from build123d import *

# Parameters (mm, degrees)
F0_R     = 11
F1_DEPTH = 7
F4_DEPTH = 0.4


with BuildPart() as f1:
    # F0 (on Front) → F1 (new body)
    with BuildSketch(Plane.XZ):
        with BuildLine():
            add(Edge.make_bspline(
                [(-90.8271871838, 17.1252166849), (-65.6361619016, 20.1801984156), (-15.2541113371, 26.2901618769), (15.053487254, 66.9980498131), (30.2072865496, 87.3519937812)],
                knots=[0, 0, 0, 0, 0.5, 1, 1, 1, 1], degree=3))
            ThreePointArc((-90.8271871838, 17.1252166849), (-100.7899149472, -0.2167571218), (-90.7526889605, -17.5157193593))
            add(Edge.make_bspline(
                [(-90.7526889605, -17.5157193593), (-65.5487567691, -20.462322529), (-15.1408923865, -26.3555288685), (15.3415164695, -66.9326828214), (30.5827208975, -87.2212597979)],
                knots=[0, 0, 0, 0, 0.5, 1, 1, 1, 1], degree=3))
            ThreePointArc((30.5827208975, -87.2212597979), (50.5826746476, -87.1782482286), (60.5454024109, -69.8362744219))
            add(Edge.make_bspline(
                [(60.2444662863, 70.096043113), (50.2908494103, 46.7157233653), (30.3950343103, -0.0180945494), (50.4991257729, -46.5724539929), (60.5454024109, -69.8362744219)],
                knots=[0, 0, 0, 0, 0.5002869612, 1, 1, 1, 1], degree=3))
            ThreePointArc((60.2444662863, 70.096043113), (50.2072402996, 87.3950053505), (30.2072865496, 87.3519937812))
        make_face()
        with Locations((-80.7899611971, -0.1737455525)):
            Circle(F0_R, mode=Mode.SUBTRACT)
        with Locations((40.5454486609, -69.8792859912)):
            Circle(F0_R, mode=Mode.SUBTRACT)
        with BuildLine():
            add(Edge.make_bspline(
                [(-11, -14), (-13.6210738364, -9.4558803164), (-8.3789261636, 0), (-16.9662275077, 15.4899287121), (4.2288329874, 25.2994830421), (11, 20)],
                knots=[0, 0, 0, 0, 0.1601841539, 0.3203683079, 0.5248038347, 0.5248038347, 0.5248038347, 0.5248038347], degree=3))
            add(Edge.make_bspline(
                [(11, 20), (19.9679398291, 12.9812032463), (19.9679398291, -12.9812032463), (11, -20)],
                knots=[0.5248038347, 0.5248038347, 0.5248038347, 0.5248038347, 0.7955644732, 0.7955644732, 0.7955644732, 0.7955644732], degree=3))
            add(Edge.make_bspline(
                [(11, -20), (4.2288329874, -25.2994830421), (-7.6548463287, -19.7994469409), (-11, -14)],
                knots=[0.7955644732, 0.7955644732, 0.7955644732, 0.7955644732, 1, 1, 1, 1], degree=3))
        make_face(mode=Mode.SUBTRACT)
        with Locations((40.2445125363, 70.0530315437)):
            Circle(F0_R, mode=Mode.SUBTRACT)
        with BuildLine():
            Line((11, 20), (11, 0))
            Line((11, 0), (11, -20))
            add(Edge.make_bspline(
                [(11, 20), (19.9679398291, 12.9812032463), (19.9679398291, -12.9812032463), (11, -20)],
                knots=[0.5248038347, 0.5248038347, 0.5248038347, 0.5248038347, 0.7955644732, 0.7955644732, 0.7955644732, 0.7955644732], degree=3))
        make_face()
    extrude(amount=F1_DEPTH)

    # F3 (on offset) → F4 (cut, symmetric)
    with BuildSketch(Plane.XZ.offset(4.5)):
        Polygon((-28.5066514462, 9.5), (-28.5066514462, 0), (-28.5066514462, -9.5), (-9.7575942054, -9.85), (-9.7575942054, 0), (-9.7575942054, 9.85), align=None)
    extrude(amount=F4_DEPTH, both=True, mode=Mode.SUBTRACT)


solid = f1.part
Build history of the part. All positions in model axes, mm. A direction names the side the tool comes from. Coordinates: 2 decimals unless noted, no trailing zeros. Write each question's results on one line, items separated by ' | '. Start each with the question number.
Item 1: Band-saw the part on A-A on x = 46. State how many separate pieces and enclosed holes the cut face has, and give its area (3 significant figures).
Item 2: Wall check: probe 1 along X at (y, z) = (-3.75, 0); probe 2 along Z at (x, y) = (36.5, -2); probe 3 along X at (y, z) = (-1.5, 3.5). Give the ranges that are in metal, low to high. Write a range as [from, to].
Item 3: Mould opens along Y. For faces 1 (the face through (-20, -4.9, 0)), 2 (the face through (45.32, -3.451, 60.294)), 3 (the face through (17, 0, 1)) say: released by +Y, released by -Y, zero draft, split by the parting line, or undercut.
Item 4: Tool access for faces 4 (the face through (-20, -4.1, 0)), 5 (the face through (50.46, -3.451, 87.247)), 6 (the face through (11, -3, 0)): list every direction of +Z, -Z, +X, -X, +Y, -Y with a clear straight run to the whole face (end or side of a thin tool).
Item 5: Flat gauge pins, fed straight in: pin 1 (2 mm diameter, centred on y = -3, z = 2.5, fed in from -X); pin 2 (4 mm diameter, centred on y = -5.5, z = 2, fed in from +X); pin 3 (1 mm diameter, centred on x = 12, y = -3, fed in from +Z); pin 4 (3 mm diameter, centred on x = -68.5, z = -22, fed in from +Y). Where does each tip first touch, or does it go through?
Numbers:
1) separate pieces: 4 | enclosed holes: 0 | area: 522 mm^2
2) probe 1: [-100.79, -91.79], [-69.79, -11], [11, 40.4] | probe 2: [-89.47, -80.11], [-59.65, 59.71], [80.4, 89.7] | probe 3: [-100.45, -91.16], [-70.42, -11.36], [11, 40.46]
3) face 1: undercut | face 2: zero draft | face 3: released by +Y
4) face 4: none | face 5: +Z, +Y, -Y | face 6: +Y, -Y
5) pin 1: x = -100.72 | pin 2: x = 40.48 | pin 3: z = 64.43 | pin 4: through
